from build123d import *

# Parameters (mm, degrees)
SKETCH_1_R          = 60
SKETCH_1_R_2        = 1.5
EXTRUDE_1_DEPTH     = 2
SKETCH_2_R          = 4
SKETCH_2_R_2        = 1.5
CUT_EXTRUDE_1_DEPTH = 2
SKETCH_3_R          = 2
CUT_EXTRUDE_2_DEPTH = 10


with BuildPart() as part:
    # 草图1 → 凸台-拉伸1 (new body)
    with BuildSketch(Plane(origin=(0, 0, 0), x_dir=(1, 0, 0), z_dir=(0, 1, 0))):
        with Locations(Location((0, 0, 0), (0, 0, 270))):
            Circle(SKETCH_1_R)
        with Locations(Location((0, 31, 0), (0, 0, 270))):
            Circle(SKETCH_1_R_2, mode=Mode.SUBTRACT)
        with Locations(Location((26.846787517, -15.5, 0), (0, 0, 270))):
            Circle(SKETCH_1_R_2, mode=Mode.SUBTRACT)
        with Locations(Location((-26.846787517, -15.5, 0), (0, 0, 270))):
            Circle(SKETCH_1_R_2, mode=Mode.SUBTRACT)
    extrude(amount=EXTRUDE_1_DEPTH)

    # 草图2 → 切除-拉伸1 (cut)
    with BuildSketch(Plane(origin=(0, 2, 0), x_dir=(1, 0, 0), z_dir=(0, 1, 0))):
        with Locations(Location((0, 0, 0), (0, 0, 270))):
            Circle(SKETCH_2_R)
        with Locations(Location((0, 7, 0), (0, 0, 270))):
            Circle(SKETCH_2_R_2)
        with Locations(Location((7, 0, 0), (0, 0, 270))):
            Circle(SKETCH_2_R_2)
        with Locations(Location((0, -7, 0), (0, 0, 270))):
            Circle(SKETCH_2_R_2)
        with Locations(Location((-7, 0, 0), (0, 0, 270))):
            Circle(SKETCH_2_R_2)
    extrude(amount=-CUT_EXTRUDE_1_DEPTH, mode=Mode.SUBTRACT)

    # 草图3 → 切除-拉伸2 (cut)
    with BuildSketch(Plane(origin=(0, 2, 0), x_dir=(1, 0, 0), z_dir=(0, 1, 0))):
        with Locations(Location((0, 55, 0), (0, 0, 270))):
            Circle(SKETCH_3_R)
        with Locations(Location((55, 0, 0), (0, 0, 270))):
            Circle(SKETCH_3_R)
        with Locations(Location((0, -55, 0), (0, 0, 270))):
            Circle(SKETCH_3_R)
        with Locations(Location((-55, 0, 0), (0, 0, 270))):
            Circle(SKETCH_3_R)
    extrude(amount=-CUT_EXTRUDE_2_DEPTH, mode=Mode.SUBTRACT)


solid = part.part
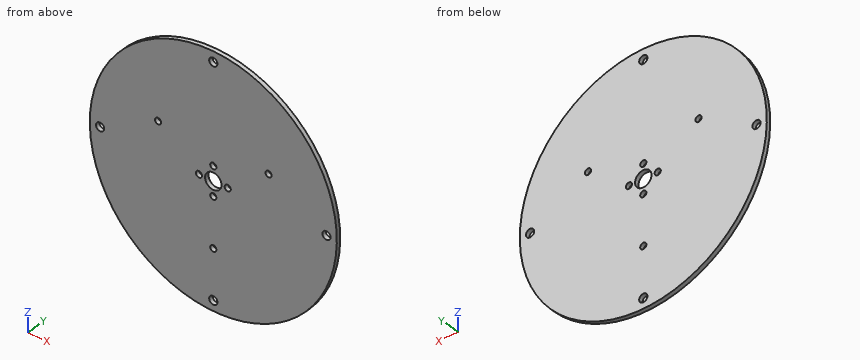
Read the model definition and answer for the solid it produces. Units are mm, in the model's axes. Give positions to 0.01 mm unless a question says otherwise; leave off trailing zeros. Write each loop counter-clockwise with the first axis right and the second up, starting at its lowest first coordinate (ties: lowest second). Pieces come first, ordered by that corner, then holes. Notation, with made-up numbers: (49.25, 68) - (82.25, 68) arc R21 cw to (82.25, 75) - close; hole circle Ø1 at (63, 78). An arc over 180 degrees is marked (long way). Answer in a Markdown table with one row per item. Add a question column.
Item 1: Flat-ended cylindrical pins translate along their axes: P1, Ø1.5, axis at x = -11, z = 28, coming from the -Y side; P2, Ø1, axis at y = 1, z = -5, coming from the -X side. Find the tip coordinate at first contact, or state that the pin passes through.
Item 2: Section A-A, the plane z = 7 is taken. Write down the section's boundary in (x, y), and give its area (3 significant figures).
Item 3: Find the intervals of material crossed by L1, parallel to X at y = 1.1, z = 0; L2, parallel to X at y = 0.5, z = 15.5; L3, parallel to X at y = 0.55, z = -55, in increasing order.
Item 4: Section C-C, the plane x = 55 is taken. Write down the section's boundary in (y, z).
Item 5: Section B-B, the plane y = 1.45 is taken. Count the separate pieces of the cut face and the enclosed holes in it, and give its area (3 significant figures).
Item 6: Section D-D, the plane x = 14.5 is taken. Write down the section's boundary in (y, z), and give its area (3 significant figures).
Recorded:
| question | item | result |
|---|---|---|
| 1 | P1 | stops at y = 0 |
| 1 | P2 | stops at x = -59.83 |
| 2 | outline | (-59.59, 0) - (-1.5, 0) - (-1.5, 2) - (-59.59, 2) - close; (1.5, 0) - (59.59, 0) - (59.59, 2) - (1.5, 2) - close |
| 2 | area | 232 mm2 |
| 3 | L1 | x = -60 to -57, -53 to -8.5, -5.5 to -4, 4 to 5.5, 8.5 to 53, 57 to 60 |
| 3 | L2 | x = -57.96 to -28.35, -25.35 to 25.35, 28.35 to 57.96 |
| 3 | L3 | x = -23.98 to -2, 2 to 23.98 |
| 4 | outline | (0, -23.98) - (2, -23.98) - (2, -2) - (0, -2) - close; (0, 2) - (2, 2) - (2, 23.98) - (0, 23.98) - close |
| 5 | separate pieces | 1 |
| 5 | enclosed holes | 12 |
| 5 | area | 11,200 mm2 |
| 6 | outline | (0, -58.22) - (2, -58.22) - (2, 58.22) - (0, 58.22) - close |
| 6 | area | 233 mm2 |
